Verification items for this drawing (mm, ordinates from the low corner). Give positions to 0.01 mm unless a question says otherwise; leave off trailing zeros. Loops run counter-clockwise (first coordinate to the right, second up) from the corner with the lowest first, then second, coordinate; pieces in that order, holes last. Notation, with made-up numbers: (43, 73) -> (97, 73) arc R6 cw to (97, 78) -> close; hole circle Ø5 at (-25, 21.25). An arc over 180 degrees is marked (long way). Write item = value, one per line.
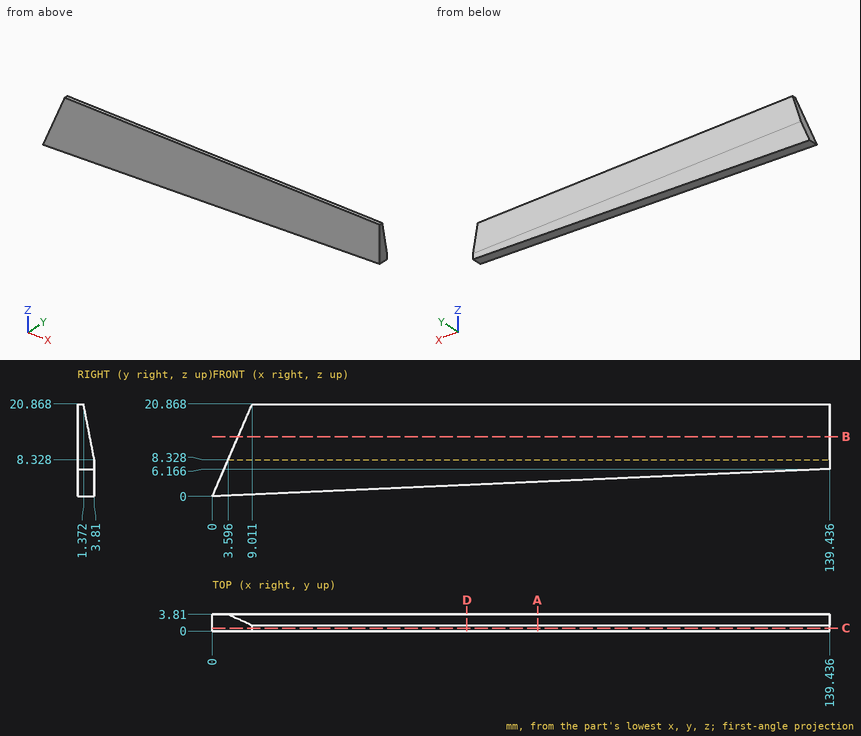
Item 1: Section check D-D, the plane x = 57.5. Record the cut outline in (y, z).
Answer:
outline = (0, 2.54) -> (3.81, 2.54) -> (3.81, 8.33) -> (1.37, 20.87) -> (0, 20.87) -> close
Item 2: Thickness scan on L1, parallel to Y at x = 90, z = 19.25; L2, parallel to Y at x = 95.5, z = 13.75 (1 decimal); L3, parallel to X at y = 1.9, z = 9.25 (1 decimal). Record the ranges inside material, lowest first. Write a range as [from, to].
Answer:
L1 = [0, 1.69]
L2 = [0, 2.8]
L3 = [4, 139.4]
Item 3: Gauge pin test, flat ends, axial feed: pin 1 (10 mm diameter, centred on x = 73.5, z = 10, fed in from -Y); pin 2 (2 mm diameter, centred on x = 49, y = 1.5, fed in from -Z); pin 3 (3 mm diameter, centred on x = 38, z = 12.5, fed in from +Y). Record the tip position at first contact, or that the pin passes through.
Answer:
pin_1 = 0
pin_2 = 2.12
pin_3 = 3.29
Item 4: Section check C-C, the plane y = 0.7. Record the cut outline in (x, z) (1 decimal).
Answer:
outline = (0, 0) -> (139.4, 6.2) -> (139.4, 20.9) -> (9, 20.9) -> close
Item 5: Section check B-B, the plane z = 13.5. Record the cut outline in (x, y) (1 decimal).
Answer:
outline = (5.8, 0) -> (139.4, 0) -> (139.4, 2.8) -> (5.8, 2.8) -> close
Item 6: Section check A-A, the plane x = 73.5. Record the cut outline in (y, z).
Answer:
outline = (0, 3.25) -> (3.81, 3.25) -> (3.81, 8.33) -> (1.37, 20.87) -> (0, 20.87) -> close
